The listing builds one solid part. Answer for the finished solid, in the listing's coordinates (mm). Face numbers are marked on the shaded views. A direction names the side the tool comes from. Coordinates: 2 decimals unless noted, no trailing zeros. Write each loop counter-clockwise with the first axis right and the second up, starting at its lowest first coordinate (ties: lowest second). Pieces come first, ordered by that corner, then holes.
from build123d import *

# Parameters (mm, degrees)
ESBO_O2_R                = 5
RESSALTO_EXTRUS_O1_DEPTH = 22.65
ESBO_O3_R                = 0.5
RESSALTO_EXTRUS_O2_DEPTH = 4.7
ESBO_O4_R                = 1
RESSALTO_EXTRUS_O3_DEPTH = 0.5
FILETE1_R                = 0.2


with BuildPart() as part:
    # Esboço2 → Ressalto-extrusão1 (new body)
    with BuildSketch(Plane(origin=(0, 0, 0), x_dir=(0, 0, -1), z_dir=(1, 0, 0))):
        Circle(ESBO_O2_R)
    extrude(amount=-RESSALTO_EXTRUS_O1_DEPTH)

    # Esboço3 → Ressalto-extrusão2 (add)
    with BuildSketch(Plane.ZY.offset(22.65)):
        with Locations(Location((0, 0, 0), (0, 0, 180))):
            Circle(ESBO_O3_R)
    extrude(amount=RESSALTO_EXTRUS_O2_DEPTH)

    # Esboço4 → Ressalto-extrusão3 (add)
    with BuildSketch(Plane.ZY.offset(22.65)):
        with Locations(Location((0, 0, 0), (0, 0, 180))):
            Circle(ESBO_O4_R)
    extrude(amount=RESSALTO_EXTRUS_O3_DEPTH)

    # Filete1
    filete1_edges = [part.edges().sort_by_distance(p)[0] for p in [
        (-22.65, 0, 5),
    ]]
    fillet(filete1_edges, radius=FILETE1_R)


solid = part.part
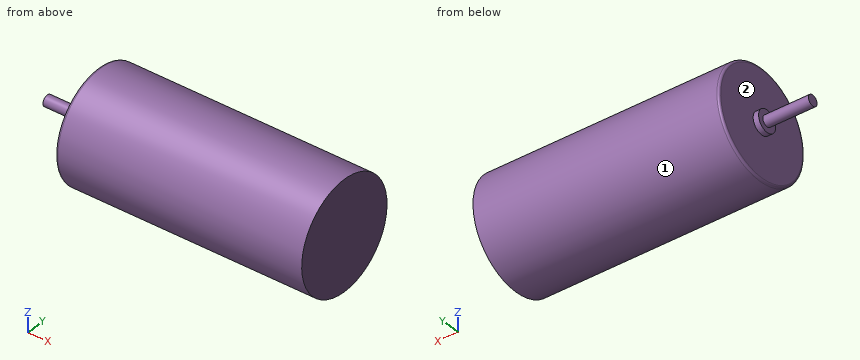
1. Find the intervals of material crossed by L1, parallel to X at y = 2.25, z = 2.5; L2, parallel to Z at x = -14.75, y = 0.25; L3, parallel to Y at x = -1, z = 4.5, in increasing order.
Results found:
L1: x = -22.65 to 0
L2: z = -4.99 to 4.99
L3: y = -2.18 to 2.18
2. Section A-A on y = 0 is taken. Give the vertices of the cut face in (x, z).
Results found:
outline: (-27.35, -0.5) - (-23.15, -0.5) - (-23.15, -1) - (-22.65, -1) - (-22.65, -4.8) arc R0.2 ccw to (-22.45, -5) - (0, -5) - (0, 5) - (-22.45, 5) arc R0.2 ccw to (-22.65, 4.8) - (-22.65, 1) - (-23.15, 1) - (-23.15, 0.5) - (-27.35, 0.5) - close
3. Section D-D on x = -24.5 is taken. Give the vertices of the cut face in (y, z).
Results found:
outline: circle Ø1 at (0, 0)
4. Flat-ended cylindrical pins translate along their axes: P1, Ø1.5, axis at y = -2, z = 3.5, coming from the -X side; P2, Ø2, axis at x = -7.5, z = 1.5, coming from the +Y side. Find the tip coordinate at first contact, or state that the pin passes through.
Results found:
P1: stops at x = -22.65
P2: stops at y = 4.97
5. Section C-C on x = -17 is taken. Give the vertices of the cut face in (y, z), then the cut area to 3 significant figures.
Results found:
outline: circle Ø10 at (0, 0)
area: 78.5 mm2
6. A tool of negligible diameter and unlimited length cuts with its end or side. For the marked faces 1 and 2, from which of +Z, -Z, +X, -X, +Y, -Y can it reach the whole face along a straight path? Write none if from no direction.
Results found:
face 1: +X, -X
face 2: -X
